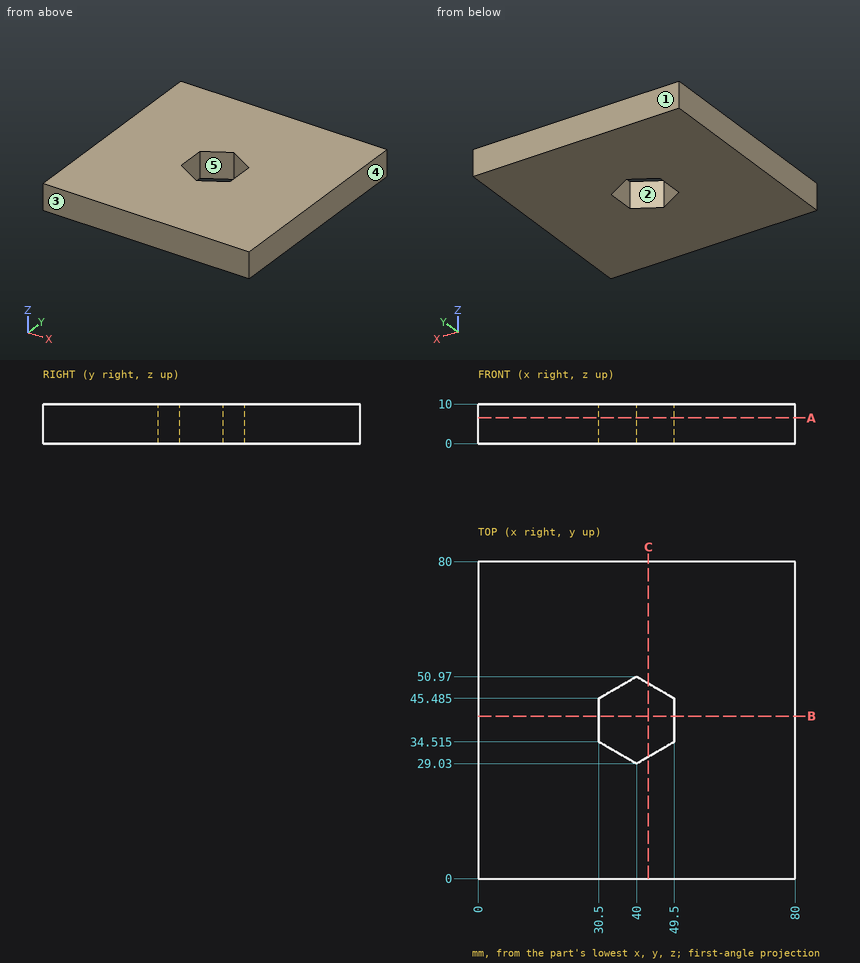
Geometry check sheet. Reference: drawing and pictorial views, mm from the part's lowest x, y, z. A direction names the side the tool comes from. Give positions to 0.01 mm unless a question says otherwise; leave off trailing zeros. Write each loop counter-clockwise with the first axis right and the second up, starting at its lowest first coordinate (ties: lowest second). Pieces come first, ordered by that corner, then holes. Notation, with made-up numbers: M 1,59.5 L 5,59.5 A16 cw 5,89.5 Z; hole C 42.25,30 d8. An arc over 180 degrees is marked long. Answer as CSV lines item,"result". Start each with the question number.
Q1. Release check for a two-part mould opening along Y. For the marked faces 3, 4 and 5 record: pulls with the +Y half, pulls with the -Y half, needs draft (parallel to the pull), parting line crosses it, or undercut.
Q2. Tool access check on the marked faces 1 and 2. Record the directions out of +Z, -Z, +X, -X, +Y, -Y that give a thin tool (end or side, any length) a straight path to the whole face; none if there is none.
Q3. Section check C-C, the plane x = 43. Record the cut outline in (y, z).
Q4. Section check A-A, the plane z = 6.5. Record the cut outline in (x, y) (1 decimal).
Q5. Material ranges on L1, parallel to X at y = 39.5, z = 3.25; L2, parallel to X at y = 30.5, z = 6 (1 decimal); L3, parallel to Y at x = 31.5, z = 6.25, recorded low to high.
Q6. Go/stop test with a flat-tipped pin: pin 1 (3 mm diameter, centred on x = 61.5, y = 49, fed in from -Z). Record where the tip stops, or that it passes through.
Q7. Section check B-B, the plane y = 41. Record the cut outline in (x, z), then the cut area to 3 significant figures.
Geometry says:
1,face 3,"pulls with the -Y half"
1,face 4,"needs draft"
1,face 5,"undercut"
2,face 1,"+Z, -Z, +X, -X, +Y"
2,face 2,"+Z, -Z"
3,outline,"M 0,0 L 30.76,0 L 30.76,10 L 0,10 Z; M 49.24,0 L 80,0 L 80,10 L 49.24,10 Z"
4,outline,"M 0,0 L 80,0 L 80,80 L 0,80 Z; hole M 30.5,34.5 L 40,29 L 49.5,34.5 L 49.5,45.5 L 40,51 L 30.5,45.5 Z"
5,L1,"0 to 30.5, 49.5 to 80"
5,L2,"0 to 37.5, 42.5 to 80"
5,L3,"0 to 33.94, 46.06 to 80"
6,pin 1,"z = 0"
7,outline,"M 0,0 L 30.5,0 L 30.5,10 L 0,10 Z; M 49.5,0 L 80,0 L 80,10 L 49.5,10 Z"
7,area,"610 mm^2"
